Verification items for the finished model (mm, model axes). Give positions to 0.01 mm unless a question says otherwise; leave off trailing zeros. Loops run counter-clockwise (first coordinate to the right, second up) from the corner with the lowest first, then second, coordinate; pieces in that order, holes last. Notation, with made-up numbers: (75, 59.25) - (104, 59.25) arc R28 cw to (104, 88.25) - close; hole circle Ø11 at (5, 11.25). An arc over 180 degrees is marked (long way). One line per item, written item: value. Start each with the question number.
1. Sectioned sample at B-B (x = 6.35). Record the cut outline in (y, z), plus the area to 3 significant figures.
2. Mould release check, pull along Y, two halves, no side actions. Record for faces 1 (the cylindrical face through (5.965, 68.114, -0.789)), 2 (the flat face through (81, 39, -1.6)): pulls with the +Y half, pulls with the -Y half, needs draft (parallel to the pull), parting line crosses it, or undercut.
3. Scan lines: L1, parallel to X at y = 69.85, z = -0.85; L2, parallel to Y at x = 82.55, z = -0.85. Record each from-to range of solid material in increasing order. Write a range as [from, to].
4. Sectioned sample at A-A (y = 69.85). Record the cut outline in (x, z), plus the area to 3 significant figures.
from build123d import *

# Parameters (mm, degrees)
SKETCH1_W          = 165.1
SKETCH1_H          = 76.2
EXTRUDE1_DEPTH     = 1.6002
SKETCH2_R          = 1.778
CUT_EXTRUDE1_DEPTH = 2.54


with BuildPart() as part:
    # Sketch1 → Extrude1 (new body)
    with BuildSketch(Plane.XY):
        with Locations((82.55, 38.1)):
            Rectangle(SKETCH1_W, SKETCH1_H)
    extrude(amount=-EXTRUDE1_DEPTH)

    # Sketch2 → Cut-Extrude1 (cut)
    with BuildSketch(Plane.XY):
        with Locations((6.35, 69.85)):
            Circle(SKETCH2_R)
        with Locations((158.75, 69.85)):
            Circle(SKETCH2_R)
        with Locations((158.75, 6.35)):
            Circle(SKETCH2_R)
        with Locations((6.35, 6.35)):
            Circle(SKETCH2_R)
        with Locations((82.55, 6.35)):
            Circle(SKETCH2_R)
        with Locations((82.55, 69.85)):
            Circle(SKETCH2_R)
    extrude(amount=-CUT_EXTRUDE1_DEPTH, mode=Mode.SUBTRACT)


solid = part.part
Results are:
1. outline: (0, -1.6) - (4.57, -1.6) - (4.57, 0) - (0, 0) - close; (8.13, -1.6) - (68.07, -1.6) - (68.07, 0) - (8.13, 0) - close; (71.63, -1.6) - (76.2, -1.6) - (76.2, 0) - (71.63, 0) - close
1. area: 111 mm^2
2. face 1: undercut
2. face 2: needs draft
3. L1: x = [0, 4.57], [8.13, 80.77], [84.33, 156.97], [160.53, 165.1]
3. L2: y = [0, 4.57], [8.13, 68.07], [71.63, 76.2]
4. outline: (0, -1.6) - (4.57, -1.6) - (4.57, 0) - (0, 0) - close; (8.13, -1.6) - (80.77, -1.6) - (80.77, 0) - (8.13, 0) - close; (84.33, -1.6) - (156.97, -1.6) - (156.97, 0) - (84.33, 0) - close; (160.53, -1.6) - (165.1, -1.6) - (165.1, 0) - (160.53, 0) - close
4. area: 247 mm^2
